The model under review builds one solid part; all positions refer to its coordinate system, in mm. A direction names the side the tool comes from. Give positions to 0.01 mm unless a question says otherwise; leave off trailing zeros. Order: outer loops, then holes, each group sorted by start corner. A loop starts at its lowest first (then second) coordinate and runs counter-clockwise, first axis right, second up. Notation, with made-up numbers: (62, 80) - (96, 80) arc R8 cw to (96, 84) - close; hole circle Ø11 at (18, 2.5). An arc over 180 degrees is marked (long way). Use CSV: the item, a comma, the result in double quotes. Start each with the question number.
```python
from build123d import *

# Parameters (mm, degrees)
ESQUISSE1_W             = 46
ESQUISSE1_H             = 73
ESQUISSE1_R             = 9.5
BOSS_EXTRU_1_DEPTH      = 5
ESQUISSE2_R             = 1.5
ESQUISSE2_W             = 5
ESQUISSE2_H             = 10
ESQUISSE2_H_2           = 5
ESQUISSE2_H_3           = 15
ENL_V_MAT_EXTRU_1_DEPTH = 5
ESQUISSE3_W             = 15.5
ESQUISSE3_H             = 5
BOSS_EXTRU_2_DEPTH      = 5


with BuildPart() as part:
    # Esquisse1 → Boss.-Extru.1 (new body)
    with BuildSketch(Plane.XY):
        with Locations((23, 36.5)):
            Rectangle(ESQUISSE1_W, ESQUISSE1_H)
        with Locations((23, 31.275)):
            Circle(ESQUISSE1_R, mode=Mode.SUBTRACT)
    extrude(amount=BOSS_EXTRU_1_DEPTH)

    # Esquisse2 → Enlèv. mat.-Extru.1 (cut)
    with BuildSketch(Plane.XY.offset(5)):
        with Locations((23, 44.275)):
            Circle(ESQUISSE2_R)
        with Locations((36, 31.275)):
            Circle(ESQUISSE2_R)
        with Locations((23, 18.275)):
            Circle(ESQUISSE2_R)
        with Locations((10, 31.275)):
            Circle(ESQUISSE2_R)
        with Locations((43.5, 58)):
            Rectangle(ESQUISSE2_W, ESQUISSE2_H)
        with Locations((2.5, 70.5)):
            Rectangle(ESQUISSE2_W, ESQUISSE2_H_2)
        with Locations((43.5, 15)):
            Rectangle(ESQUISSE2_W, ESQUISSE2_H)
        with Locations((2.5, 15)):
            Rectangle(ESQUISSE2_W, ESQUISSE2_H)
        with Locations((2.5, 55.5)):
            Rectangle(ESQUISSE2_W, ESQUISSE2_H_3)
        with Locations((43.5, 70.5)):
            Rectangle(ESQUISSE2_W, ESQUISSE2_H_2)
        with Locations((23, 70.5)):
            Rectangle(ESQUISSE2_W, ESQUISSE2_H_2)
    extrude(amount=-ENL_V_MAT_EXTRU_1_DEPTH, mode=Mode.SUBTRACT)

    # Esquisse3 → Boss.-Extru.2 (add)
    with BuildSketch(Plane(origin=(0, 0, 0), x_dir=(-1, 0, 0), z_dir=(0, 0, -1))):
        with Locations((-33.25, 75.5)):
            Rectangle(ESQUISSE3_W, ESQUISSE3_H)
        with Locations((-12.75, 75.5)):
            Rectangle(ESQUISSE3_W, ESQUISSE3_H)
        with Locations((-33.25, -2.5)):
            Rectangle(ESQUISSE3_W, ESQUISSE3_H)
        with Locations((-12.75, -2.5)):
            Rectangle(ESQUISSE3_W, ESQUISSE3_H)
    extrude(amount=-BOSS_EXTRU_2_DEPTH)


solid = part.part
```
1. Clearance check with flat-ended pins moving along their axes: pin 1 (1.5 mm diameter, centred on y = -3.5, z = 2.5, fed in from +X); pin 2 (2.5 mm diameter, centred on x = 42.5, z = 3, fed in from -Y); pin 3 (2.5 mm diameter, centred on y = 12.5, z = 3.5, fed in from -X). State where each tip first meets the part, or that it passes through.
2. Consider section D-D (y = 58.5). Give the boundary of the cut face in (x, z).
3. To check wall thickness, follow L1, parallel to Y at x = 23, z = 3.35 (3 decimals); L2, parallel to X at y = 54, z = 3.65; L3, parallel to Y at x = 36, z = 3.5 (3 decimals). State the ranges of each line that lie inside material, in increasing order. Write a range as [from, to].
4. Mouldability with a two-part tool opening along X and no side actions: class faces 5 (the face through (41, 15, 3)), 6 (the face through (31.776, 27.636, 2.465)), 7 (the face through (5, 55, 3)) as pulls with the +X half, pulls with the -X half, needs draft (parallel to the pull), parting line crosses it, or undercut.
5. Tool access review of faces 1 (the face through (43, 68, 3)), 2 (the face through (2, 20, 3)), 3 (the face through (5, -3, 2)), 4 (the face through (20.5, -3, 2)): name each direction out of +Z, -Z, +X, -X, +Y, -Y from which nothing blocks a thin tool from reaching the whole face with its end or side.
6. Consider section B-B (x = 36). Give the boundary of the cut face in (y, z) (3 decimals).
7. Consider section A-A (x = 23). Give the boundary of the cut face in (y, z) (3 decimals).
8. Consider section C-C (y = 24). Give the boundary of the cut face in (x, z), and give its area (3 significant figures).
Answers follow:
1,pin 1,"stops at x = 41"
1,pin 2,"stops at y = 0"
1,pin 3,"stops at x = 5"
2,outline,"(5, 0) - (41, 0) - (41, 5) - (5, 5) - close"
3,L1,"y = [0, 16.775], [19.775, 21.775], [40.775, 42.775], [45.775, 68]"
3,L2,"x = [5, 41]"
3,L3,"y = [-5, 29.775], [32.775, 78]"
4,face 5,"pulls with the +X half"
4,face 6,"undercut"
4,face 7,"pulls with the -X half"
5,face 1,"+Z, -Z, +X, +Y"
5,face 2,"+Z, -Z, -X"
5,face 3,"+Z, -Z, -X, -Y"
5,face 4,"+Z, -Z, -Y"
6,outline,"(-5, 0) - (29.775, 0) - (29.775, 5) - (-5, 5) - close; (32.775, 0) - (78, 0) - (78, 5) - (32.775, 5) - close"
7,outline,"(0, 0) - (16.775, 0) - (16.775, 5) - (0, 5) - close; (19.775, 0) - (21.775, 0) - (21.775, 5) - (19.775, 5) - close; (40.775, 0) - (42.775, 0) - (42.775, 5) - (40.775, 5) - close; (45.775, 0) - (68, 0) - (68, 5) - (45.775, 5) - close"
8,outline,"(0, 0) - (16.89, 0) - (16.89, 5) - (0, 5) - close; (29.11, 0) - (46, 0) - (46, 5) - (29.11, 5) - close"
8,area,"169 mm^2"
